from build123d import *

# Parameters (mm, degrees)
SKETCH1_R           = 3.175
SKETCH1_W           = 562.160000372
SKETCH1_H           = 153.482
BOSS_EXTRUDE1_DEPTH = 76.2
CUT_EXTRUDE1_REACH  = 662.854


with BuildPart() as part:
    # Sketch1 → Boss-Extrude1 (new body)
    with BuildSketch(Plane(origin=(0, 0, 0), x_dir=(1, 0, 0), z_dir=(0, 1, 0))):
        with BuildLine():
            Line((-514.30312852, -129.851740003), (-1083.763128892, -129.851740003))
            ThreePointArc((-1083.763128892, -129.851740003), (-1088.253256953, -131.711611942), (-1090.113128892, -136.201740003))
            Line((-1090.113128892, -136.201740003), (-1090.113128892, -296.983740003))
            ThreePointArc((-1090.113128892, -296.983740003), (-1088.253256953, -301.473868063), (-1083.763128892, -303.333740003))
            Line((-1083.763128892, -303.333740003), (-514.30312852, -303.333740003))
            ThreePointArc((-514.30312852, -303.333740003), (-509.81300046, -301.473868063), (-507.95312852, -296.983740003))
            Line((-507.95312852, -296.983740003), (-507.95312852, -136.201740003))
            ThreePointArc((-507.95312852, -136.201740003), (-509.81300046, -131.711611942), (-514.30312852, -129.851740003))
        make_face()
        with Locations(Location((-1083.763128892, -136.201740003, 0), (0, 0, 90))):
            Circle(SKETCH1_R, mode=Mode.SUBTRACT)
        with Locations(Location((-1083.763128892, -296.983740003, 0), (0, 0, 90))):
            Circle(SKETCH1_R, mode=Mode.SUBTRACT)
        with Locations(Location((-514.30312852, -136.201740003, 0), (0, 0, 90))):
            Circle(SKETCH1_R, mode=Mode.SUBTRACT)
        with Locations(Location((-514.30312852, -296.983740003, 0), (0, 0, 90))):
            Circle(SKETCH1_R, mode=Mode.SUBTRACT)
        with Locations((-799.033128706, -216.592740003)):
            Rectangle(SKETCH1_W, SKETCH1_H, mode=Mode.SUBTRACT)
    extrude(amount=BOSS_EXTRUDE1_DEPTH)

    # Sketch3 → Cut-Extrude1 (cut, up to next)
    with BuildSketch(Plane.ZY.offset(1090.113128892), mode=Mode.PRIVATE) as cut_extrude1_sk1:
        with BuildLine():
            Line((161.601740003, 0), (148.901740003, 0))
            Line((148.901740003, 0), (148.901740003, 12.7))
            ThreePointArc((148.901740003, 12.7), (155.251740003, 19.05), (161.601740003, 12.7))
            Line((161.601740003, 12.7), (161.601740003, 0))
        make_face()
    cut_extrude1_tool1 = extrude(cut_extrude1_sk1.sketch, amount=-CUT_EXTRUDE1_REACH, mode=Mode.PRIVATE) & part.part
    # Sketch3 → Cut-Extrude1 (cut, up to next)
    with BuildSketch(Plane.ZY.offset(1090.113128892), mode=Mode.PRIVATE) as cut_extrude1_sk2:
        with BuildLine():
            Line((199.701740003, 0), (187.001740003, 0))
            Line((187.001740003, 0), (187.001740003, 12.7))
            ThreePointArc((187.001740003, 12.7), (193.351740003, 19.05), (199.701740003, 12.7))
            Line((199.701740003, 12.7), (199.701740003, 0))
        make_face()
    cut_extrude1_tool2 = extrude(cut_extrude1_sk2.sketch, amount=-CUT_EXTRUDE1_REACH, mode=Mode.PRIVATE) & part.part
    # Sketch3 → Cut-Extrude1 (cut, up to next)
    with BuildSketch(Plane.ZY.offset(1090.113128892), mode=Mode.PRIVATE) as cut_extrude1_sk3:
        with BuildLine():
            Line((237.801740003, 0), (225.101740003, 0))
            Line((225.101740003, 0), (225.101740003, 12.7))
            ThreePointArc((225.101740003, 12.7), (231.451740003, 19.05), (237.801740003, 12.7))
            Line((237.801740003, 12.7), (237.801740003, 0))
        make_face()
    cut_extrude1_tool3 = extrude(cut_extrude1_sk3.sketch, amount=-CUT_EXTRUDE1_REACH, mode=Mode.PRIVATE) & part.part
    # Sketch3 → Cut-Extrude1 (cut, up to next)
    with BuildSketch(Plane.ZY.offset(1090.113128892), mode=Mode.PRIVATE) as cut_extrude1_sk4:
        with BuildLine():
            Line((275.901740003, 0), (263.201740003, 0))
            Line((263.201740003, 0), (263.201740003, 12.7))
            ThreePointArc((263.201740003, 12.7), (269.551740003, 19.05), (275.901740003, 12.7))
            Line((275.901740003, 12.7), (275.901740003, 0))
        make_face()
    cut_extrude1_tool4 = extrude(cut_extrude1_sk4.sketch, amount=-CUT_EXTRUDE1_REACH, mode=Mode.PRIVATE) & part.part
    add(cut_extrude1_tool1.solids().sort_by_distance((-1090.113129, 8.900424, 155.25174))[0], mode=Mode.SUBTRACT)
    add(cut_extrude1_tool2.solids().sort_by_distance((-1090.113129, 8.900424, 193.35174))[0], mode=Mode.SUBTRACT)
    add(cut_extrude1_tool3.solids().sort_by_distance((-1090.113129, 8.900424, 231.45174))[0], mode=Mode.SUBTRACT)
    add(cut_extrude1_tool4.solids().sort_by_distance((-1090.113129, 8.900424, 269.55174))[0], mode=Mode.SUBTRACT)


solid = part.part
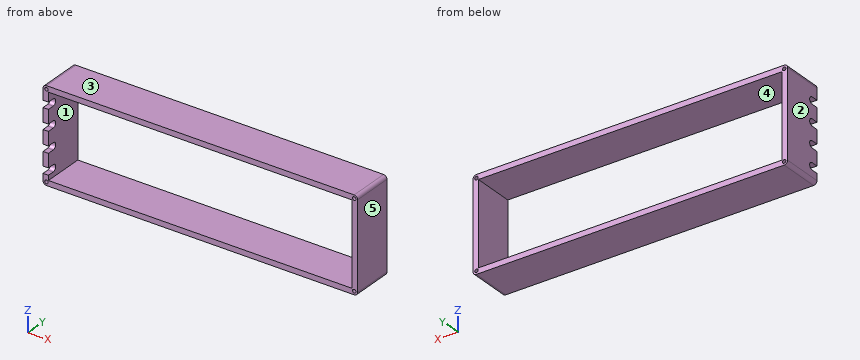
CAD build for the part. Positions are in the model's coordinates, mm. Face numbers are marked on the shaded views. A direction names the side the tool comes from. Coordinates: 2 decimals unless noted, no trailing zeros. Write each loop counter-clockwise with the first axis right and the second up, starting at its lowest first coordinate (ties: lowest second). Pieces come first, ordered by that corner, then holes. Notation, with made-up numbers: (88.5, 86.5) - (143.5, 86.5) arc R20 ccw to (143.5, 116.5) - close; hole circle Ø1 at (-27.5, 24.25). An arc over 180 degrees is marked (long way). Use a Markdown table: item, result. Add a question column.
Item 1: Mould opens along X. For the marked faces 3, 4 and 5 say: pulls with the +X half, pulls with the -X half, needs draft (parallel to the pull), parting line crosses it, or undercut.
Item 2: Band-saw the part on A-A, the plane z = 288. Give the cut face in (x, y), and give its area (3 significant figures).
Item 3: 3-axis set-ups, long thin cutter, end or side, ignore diameter. For the marked faces 1 and 2: which of +Z, -Z, +X, -X, +Y, -Y reach the whole face in a straight line?
Item 4: Band-saw the part on C-C, the plane y = 40. Give the cut face in (x, z) (3 decimals), and give its area (3 significant figures).
Item 5: Drill centre lines: L1, parallel to X at y = 33, z = 220; L2, parallel to Z at x = -965, y = 36; L3, parallel to X at y = 16, z = 154.5. Where is each one in solid material? Low to high. Write a range as from..to.
Item 6: Band-saw the part on B-B, the plane x = -863. Give the cut face in (y, z).
Item 7: Flat gauge pins, fed straight in: pin 1 (5 mm diameter, centred on x = -1086.5, y = 3.5, fed in from +Z); pin 2 (5 mm diameter, centred on x = -1086.5, y = 6.5, fed in from -Z). Where does each tip first touch, or does it go through?
Numbers:
| question | item | result |
|---|---|---|
| 1 | face 3 | needs draft |
| 1 | face 4 | undercut |
| 1 | face 5 | pulls with the +X half |
| 2 | outline | (-1090.11, 0) - (-1080.11, 0) - (-1080.11, 76.2) - (-1090.11, 76.2) - close; (-517.95, 0) - (-507.95, 0) - (-507.95, 76.2) - (-517.95, 76.2) - close |
| 2 | area | 1,520 mm2 |
| 3 | face 1 | +Y, -Y |
| 3 | face 2 | +Z, -Z, -X, +Y, -Y |
| 4 | outline | (-1090.113, 136.202) arc R6.35 ccw to (-1083.763, 129.852) - (-514.303, 129.852) arc R6.35 ccw to (-507.953, 136.202) - (-507.953, 296.984) arc R6.35 ccw to (-514.303, 303.334) - (-1083.763, 303.334) arc R6.35 ccw to (-1090.113, 296.984) - close; hole circle Ø6.35 at (-1083.763, 136.202); hole circle Ø6.35 at (-1083.763, 296.984); hole (-1080.113, 139.852) - (-517.953, 139.852) - (-517.953, 293.334) - (-1080.113, 293.334) - close; hole circle Ø6.35 at (-514.303, 136.202); hole circle Ø6.35 at (-514.303, 296.984) |
| 4 | area | 14,600 mm2 |
| 5 | L1 | -1090.11..-1080.11, -517.95..-507.95 |
| 5 | L2 | 129.85..139.85, 293.33..303.33 |
| 5 | L3 | -517.95..-507.95 |
| 6 | outline | (0, 129.85) - (76.2, 129.85) - (76.2, 139.85) - (0, 139.85) - close; (0, 293.33) - (76.2, 293.33) - (76.2, 303.33) - (0, 303.33) - close |
| 7 | pin 1 | z = 303.33 |
| 7 | pin 2 | z = 129.86 |
